```python
from build123d import *

# Parameters (mm, degrees)
CROQUIS1_R              = 6.35
SALIENTE_EXTRUIR1_DEPTH = 125
CROQUIS2_R              = 6.35
SALIENTE_EXTRUIR2_DEPTH = 40
CROQUIS3_W              = 5
CROQUIS3_H              = 5
CORTAR_EXTRUIR1_DEPTH   = 20


with BuildPart() as part:
    # Croquis1 → Saliente-Extruir1 (new, symmetric)
    with BuildSketch(Plane.XY):
        Circle(CROQUIS1_R)
    extrude(amount=SALIENTE_EXTRUIR1_DEPTH, both=True)

    # Croquis2 → Saliente-Extruir2 (add)
    with BuildSketch(Plane(origin=(0, 0, 0), x_dir=(0, 0, -1), z_dir=(1, 0, 0))):
        Circle(CROQUIS2_R)
        with Locations((110, 0)):
            Circle(CROQUIS2_R)
        with Locations((-110, 0)):
            Circle(CROQUIS2_R)
    extrude(amount=SALIENTE_EXTRUIR2_DEPTH)

    # Croquis3 → Cortar-Extruir1 (cut)
    with BuildSketch(Plane.XY.offset(125)):
        with Locations((0, -6.35)):
            Rectangle(CROQUIS3_W, CROQUIS3_H)
    extrude(amount=-CORTAR_EXTRUIR1_DEPTH, mode=Mode.SUBTRACT)


solid = part.part
```
The model under review builds one solid part; all positions refer to its coordinate system, in mm. A direction names the side the tool comes from. Give positions to 0.01 mm unless a question says otherwise; leave off trailing zeros. Write each loop counter-clockwise with the first axis right and the second up, starting at its lowest first coordinate (ties: lowest second). Pieces come first, ordered by that corner, then holes. Notation, with made-up numbers: (75, 72.5) - (126, 72.5) arc R33 cw to (126, 109.5) - close; hole circle Ø4 at (68.25, 34.25). An arc over 180 degrees is marked (long way). Answer in a Markdown table with one row per item. Add a question column.
1. Wall thickness on line 1 along Z through (x, y) = (5, 5.25); line 2 along Z through (x, y) = (22.5, -5); line 3 along Z through (x, y) = (-1.5, -5): over which ranges is each line inside the solid? List them lowest first. Write a range as [from, to].
2. We need section C-C on y = 2. Write out the cut boundary in (x, z), then the cut area to 3 significant figures.
3. Draft analysis for pull direction Z (two halves, no side actions). For faces 4 (the flat face through (40, 0, -110)), 5 (the flat face through (0, 0, 125)), 6 (the cylindrical face through (19.72, 0.279, -103.656)), state which applies: +Z half, -Z half, draft (parallel to the pull), parting line (faces both ways), or undercut.
4. Insertion check: P1, Ø0.8, axis at x = -1, y = -4.5, coming from the +Z side; P2, Ø2, axis at y = -5.5, z = 119.5, coming from the -X side; P3, Ø2.5, axis at x = 0.5, z = 115, coming from the -Y side. Each pin has a flat end and moves straight along its axis. Give the tip position at first contact, or say it passes through.
5. We need section D-D on z = -83. Write out the cut boundary in (x, y), then the cut area to 3 significant figures.
6. We need section B-B on x = 26. Write out the cut boundary in (y, z).
7. Tool access review of faces 1 (the flat face through (0, 0, -125)), 2 (the flat face through (0, -3.85, 115)), 3 (the cylindrical face through (19.7, 6.3, 110.8)): name each direction out of +Z, -Z, +X, -X, +Y, -Y from which nothing blocks a thin tool from reaching the whole face with its end or side.
8. We need section A-A on z = 110. Write out the cut boundary in (x, y), then the cut area to 3 significant figures.
Ans:
| question | item | result |
|---|---|---|
| 1 | line 1 | z = [-113.57, -106.43], [-3.57, 3.57], [106.43, 113.57] |
| 1 | line 2 | z = [-113.91, -106.09], [-3.91, 3.91], [106.09, 113.91] |
| 1 | line 3 | z = [-125, 105] |
| 2 | outline | (-6.03, -125) - (6.03, -125) - (6.03, -116.03) - (40, -116.03) - (40, -103.97) - (6.03, -103.97) - (6.03, -6.03) - (40, -6.03) - (40, 6.03) - (6.03, 6.03) - (6.03, 103.97) - (40, 103.97) - (40, 116.03) - (6.03, 116.03) - (6.03, 125) - (-6.03, 125) - close |
| 2 | area | 4,240 mm^2 |
| 3 | face 4 | draft |
| 3 | face 5 | +Z half |
| 3 | face 6 | undercut |
| 4 | P1 | stops at z = 105 |
| 4 | P2 | stops at x = -4.48 |
| 4 | P3 | stops at y = -3.85 |
| 5 | outline | circle Ø12.7 at (0, 0) |
| 5 | area | 127 mm^2 |
| 6 | outline | circle Ø12.7 at (0, -110); circle Ø12.7 at (0, 0); circle Ø12.7 at (0, 110) |
| 7 | face 1 | -Z, +X, -X, +Y, -Y |
| 7 | face 2 | +Z, -Y |
| 7 | face 3 | +X |
| 8 | outline | (-2.5, -5.84) - (-2.5, -3.85) - (2.5, -3.85) - (2.5, -6.35) - (40, -6.35) - (40, 6.35) - (0, 6.35) arc R6.35 ccw to start |
| 8 | area | 559 mm^2 |
